Can you work these out from the model? Positions are in its coordinate system, mm. A direction names the side the tool comes from. Give positions to 0.01 mm unless a question says otherwise; leave off trailing zeros. Loops run counter-clockwise (first coordinate to the right, second up) from the corner with the lowest first, then second, coordinate; pieces in that order, holes last. Notation, with made-up numbers: (16.25, -37.75) -> (53.25, -37.75) arc R23 ccw to (53.25, -19.75) -> close; hole circle Ø6 at (45.5, -17). An arc over 180 degrees is marked (long way). Use CSV: the item, a comma, the result in double quotes.
from build123d import *

# Parameters (mm, degrees)
F3_DEPTH = 3
F4_SIZE  = 0.6


with BuildPart() as f1:
    # F0 (on Front) → F1 (revolve)
    with BuildSketch(Plane.XZ):
        Polygon((3, 8), (0, 8), (0, 1.65), (15, 1.65), (15, 3.7), (18, 3.7), (18, 5.5), (3, 5.5), align=None)
    revolve(axis=Axis((6.870626, 0, 0), (1, 0, 0)))

    # F2 (on face) → F3 (cut)
    with BuildSketch(Plane(origin=(0, 0, 0), x_dir=(0, -1, 0), z_dir=(-1, 0, 0))):
        Polygon((-1.645448, -2.85), (1.645448, -2.85), (3.290897, 0), (1.645448, 2.85), (-1.645448, 2.85), (-3.290897, 0), align=None)
    extrude(amount=-F3_DEPTH, mode=Mode.SUBTRACT)

    # F4
    f4_edges = [f1.edges().sort_by_distance(p)[0] for p in [
        (0, 0, -8),
        (18, 0, -3.7),
        (15, 0, -1.65),
        (3, 0, -8),
    ]]
    chamfer(f4_edges, length=F4_SIZE)


solid = f1.part
(1) We'd pull the mould along Y, two halves only. Please class faces 4 (the face through (1.479, 2.48, -1.405)), 5 (the face through (18, 4, -2)), 6 (the face through (1.49, 7.81, -1.73)): released by +Y, released by -Y, zero draft, split by the parting line, or undercut.
Answer sheet:
face 4,"undercut"
face 5,"zero draft"
face 6,"split by the parting line"
(2) If we section it at C-C, the plane x = 16.5: Write out the boundary of the cut face in (y, z).
Answer sheet:
outline,"circle Ø11 at (0, 0); hole circle Ø7.4 at (0, 0)"
(3) If we section it at A-A, the plane y = 0: Write out the boundary of the cut face in (x, z), then the cut area to 3 significant figures.
Answer sheet:
outline,"(0, -7.4) -> (0.6, -8) -> (2.4, -8) -> (3, -7.4) -> (3, -5.5) -> (18, -5.5) -> (18, -4.3) -> (17.4, -3.7) -> (15, -3.7) -> (15, -2.25) -> (14.4, -1.65) -> (3, -1.65) -> (3, -2.85) -> (0, -2.85) -> close; (0, 2.85) -> (3, 2.85) -> (3, 1.65) -> (14.4, 1.65) -> (15, 2.25) -> (15, 3.7) -> (17.4, 3.7) -> (18, 4.3) -> (18, 5.5) -> (3, 5.5) -> (3, 7.4) -> (2.4, 8) -> (0.6, 8) -> (0, 7.4) -> close"
area,"133 mm2"
(4) If I drill on L1, parallel to Y at x = 16.9, z = 0; L2, parallel to Y at x = 5.5, z = 0, over which ranges is the centre line in solid material (lowest first)? Write a range as from..to.
Answer sheet:
L1,"y = -5.5..-3.7, 3.7..5.5"
L2,"y = -5.5..-1.65, 1.65..5.5"
(5) Will these pins go through, and if not, where does the flat tip stop? pin 1 Ø6 at (y, z) = (0, 0) entering from +X; pin 2 Ø2 at (y, z) = (-1, -0.5) entering from +X; pin 3 Ø4 at (x, y) = (11, 3.5) entering from +Z; pin 4 Ø3 at (y, z) = (0, 0) entering from +X.
Answer sheet:
pin 1,"stops at x = 15"
pin 2,"stops at x = 14.87"
pin 3,"stops at z = 5.29"
pin 4,"passes through"
(6) If we section it at B-B, the plane x = 2: Write out the boundary of the cut face in (y, z), then the cut area to 3 significant figures.
Answer sheet:
outline,"circle Ø16 at (0, 0); hole (-3.29, 0) -> (-1.65, -2.85) -> (1.65, -2.85) -> (3.29, 0) -> (1.65, 2.85) -> (-1.65, 2.85) -> close"
area,"173 mm2"
(7) If we section it at D-D, the plane x = 7: Write out the boundary of the cut face in (y, z), then the cut area to 3 significant figures.
Answer sheet:
outline,"circle Ø11 at (0, 0); hole circle Ø3.3 at (0, 0)"
area,"86.5 mm2"
(8) Which directions (+Z, -Z, +X, -X, +Y, -Y) give clear straight access to the entire face, cutting with the end or side of a thin tool? Please do faces 1 (the face through (15, 2, -2)), 2 (the face through (1.48, 2.46, 1.44)), 3 (the face through (0, -0.1, 3.2)).
Answer sheet:
face 1,"+X"
face 2,"-X"
face 3,"+Z, -Z, -X, +Y, -Y"
